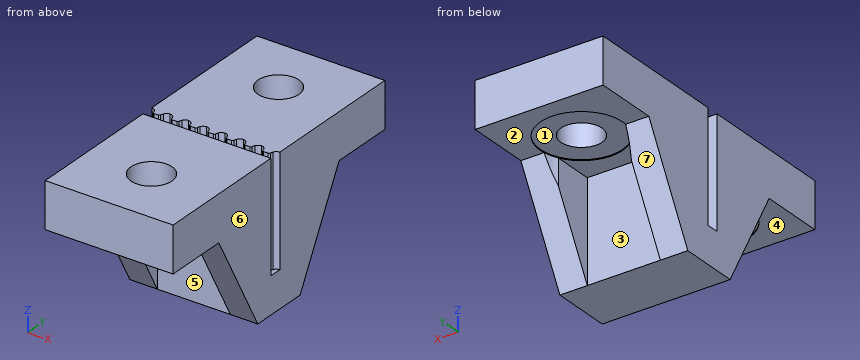
```python
from build123d import *

# Parameters (mm, degrees)
SKETCH3_W           = 14
SKETCH3_H           = 6.5
BOSS_EXTRUDE2_DEPTH = 16
CUT_EXTRUDE1_START  = 4
CUT_EXTRUDE1_DEPTH  = 19
LPATTERN2_COUNT     = 7
LPATTERN2_PITCH     = 2
SKETCH4_W           = 14
SKETCH4_H           = 13
SKETCH4_R           = 2.25
BOSS_EXTRUDE3_DEPTH = 5
BOSS_EXTRUDE4_DEPTH = 3
BOSS_EXTRUDE5_START = -11
BOSS_EXTRUDE5_DEPTH = 3
CUT_EXTRUDE2_START  = -0.1
SKETCH5_R           = 4.5
CUT_EXTRUDE2_DEPTH  = 10.1


with BuildPart() as part:
    # Sketch3 → Boss-Extrude2 (new body)
    with BuildSketch(Plane.XY):
        with Locations((7, 1.25)):
            Rectangle(SKETCH3_W, SKETCH3_H)
    extrude(amount=BOSS_EXTRUDE2_DEPTH)

    # Sketch1 → Cut-Extrude1 (cut)
    with BuildSketch(Plane.XY.offset(CUT_EXTRUDE1_START)):
        with BuildLine():
            Line((0.740175425, 0.63), (1.259824575, 0.63))
            ThreePointArc((1.259824575, 0.63), (1.358731646, 0.667228588), (1.408543109, 0.760434783))
            ThreePointArc((1.408543109, 0.760434783), (1.442388286, 0.918062154), (1.501123596, 1.068202247))
            ThreePointArc((1.501123596, 1.068202247), (1.705850588, 1.295639059), (2, 1.38))
            Line((2, 1.38), (2, 0))
            Line((2, 0), (0, 0))
            Line((0, 0), (0, 1.38))
            ThreePointArc((0, 1.38), (0.294149412, 1.295639059), (0.498876404, 1.068202247))
            ThreePointArc((0.498876404, 1.068202247), (0.557611714, 0.918062154), (0.591456891, 0.760434783))
            ThreePointArc((0.591456891, 0.760434783), (0.641268354, 0.667228588), (0.740175425, 0.63))
        make_face()
    cut_extrude1 = extrude(amount=CUT_EXTRUDE1_DEPTH, mode=Mode.SUBTRACT)

    # LPattern2: Cut-Extrude1 ×7
    with Locations(*[(i * LPATTERN2_PITCH, 0, 0) for i in range(1, LPATTERN2_COUNT)]):
        add(cut_extrude1, mode=Mode.SUBTRACT)

    # Sketch4 → Boss-Extrude3 (add)
    with BuildSketch(Plane(origin=(0, 4.5, 16), x_dir=(-1, 0, 0), z_dir=(0, 0, -1))):
        with Locations((-7, -13)):
            Rectangle(SKETCH4_W, SKETCH4_H)
        with Locations((-7, -13)):
            Circle(SKETCH4_R, mode=Mode.SUBTRACT)
        with Locations((-7, 6.5)):
            Rectangle(SKETCH4_W, SKETCH4_H)
        with Locations((-7, 6.5)):
            Circle(SKETCH4_R, mode=Mode.SUBTRACT)
    extrude(amount=BOSS_EXTRUDE3_DEPTH)

    # Sketch7 → Boss-Extrude4 (add)
    with BuildSketch(Plane.ZY):
        Polygon((0, -2), (11, -7.982839213), (11, -2), align=None)
    boss_extrude4 = extrude(amount=-BOSS_EXTRUDE4_DEPTH)

    # Sketch7_2 → Boss-Extrude5 (add)
    with BuildSketch(Plane.ZY.offset(BOSS_EXTRUDE5_START)):
        Polygon((0, -2), (11, -7.982839213), (11, -2), align=None)
    boss_extrude5 = extrude(amount=-BOSS_EXTRUDE5_DEPTH)

    # Sketch5 → Cut-Extrude2 (cut)
    with BuildSketch(Plane(origin=(0, 0, 11), x_dir=(-1, 0, 0), z_dir=(0, 0, -1)).offset(CUT_EXTRUDE2_START)):
        with Locations((-7, 11)):
            Circle(SKETCH5_R)
        with Locations((-7, -8.5)):
            Circle(SKETCH5_R)
    cut_extrude2 = extrude(amount=CUT_EXTRUDE2_DEPTH, mode=Mode.SUBTRACT)

    # Mirror1: Boss-Extrude4, Boss-Extrude5, Cut-Extrude2 across plane
    add(boss_extrude4.mirror(Plane.ZX.offset(1.25)))
    add(boss_extrude5.mirror(Plane.ZX.offset(1.25)))
    add(cut_extrude2.mirror(Plane.ZX.offset(1.25)), mode=Mode.SUBTRACT)


solid = part.part
```
The listing builds one solid part. Answer for the finished solid, in the listing's coordinates (mm). Face numbers are marked on the shaded views. A direction names the side the tool comes from. Coordinates: 2 decimals unless noted, no trailing zeros. Write each loop counter-clockwise with the first axis right and the second up, starting at its lowest first coordinate (ties: lowest second). Pieces come first, ordered by that corner, then holes. Notation, with made-up numbers: (0.5, -32.5) - (45.5, -32.5) arc R24 ccw to (45.5, -17.5) - close; hole circle Ø3 at (-10, -4.5). An arc over 180 degrees is marked (long way). Return JSON: item names as keys, results as strings. Group by question number.
Q1. The part is cut by section D-D on y = -10. Write down the section's boundary in (x, z), and give its area (3 significant figures).
Q2. Find the intervals of material crossed by line 1 along Y through (x, z) = (7, 12.7); line 2 along X through (y, z) = (7, 9); line 3 along Y through (x, z) = (7, 9.65), in increasing order. Write a range as [from, to].
Q3. Which of the six approach directions +Z, -Z, +X, -X, +Y, -Y give full straight-line access (tool end or side, diameter ignored) to the marked faces 1, 2, 3 and 4?
Q4. The part is cut by section A-A on y = 11. Write down the section's boundary in (x, z).
Q5. The part is cut by section C-C on y = -3. Write down the section's boundary in (x, z), and give its area (3 significant figures).
Q6. Flat-ended cylindrical pins translate along their axes: pin 1 Ø3.5 at (x, y) = (9, -4.5) entering from -Z; pin 2 Ø6.5 at (x, z) = (7.5, 5) entering from -Y; pin 3 Ø4 at (y, z) = (-7.5, 3) entering from -X; pin 4 Ø5 at (y, z) = (-4.5, 3) entering from -X. Find the tip coordinate at first contact, or state that the pin passes through.
Q7. The part is cut by section B-B on z = 15.25. State how many separate pieces and enclosed holes the cut face has, and give its area (3 significant figures).
Q8. For a pull along X with two mould halves and no side action, classify the marked faces 5, 6 and 7 as +X half, -X half, draft (parallel to the pull), parting line (faces both ways), or undercut.
Evaluation:
{
 "1": {"outline": "(0, 11) - (2.76, 11) - (2.76, 11.1) - (5.32, 11.1) - (5.32, 16) - (0, 16) - close; (8.68, 11.1) - (11.24, 11.1) - (11.24, 11) - (14, 11) - (14, 16) - (8.68, 16) - close", "area": "52.7 mm2"},
 "2": {"line 1": "y = [-15, -10.75], [-6.25, 0], [0.63, 8.75], [13.25, 17.5]", "line 2": "x = [0, 3], [11, 14]", "line 3": "y = [-2, 0], [0.63, 4.5]"},
 "3": {"face 1": "-Z", "face 2": "-Z, +X, -X, +Y", "face 3": "-Z, +Y", "face 4": "-Z, +X, -X, -Y"},
 "4": {"outline": "(0, 11) - (2.5, 11) - (2.5, 11.1) - (4.75, 11.1) - (4.75, 16) - (0, 16) - close; (9.25, 11.1) - (11.5, 11.1) - (11.5, 11) - (14, 11) - (14, 16) - (9.25, 16) - close"},
 "5": {"outline": "(0, 1.84) - (3, 1.84) - (3, 11) - (11, 11) - (11, 1.84) - (14, 1.84) - (14, 16) - (0, 16) - close", "area": "125 mm2"},
 "6": {"pin 1": "stops at z = 11", "pin 2": "stops at y = -2", "pin 3": "passes through", "pin 4": "stops at x = 0"},
 "7": {"separate pieces": "2", "enclosed holes": "2", "area": "409 mm2"},
 "8": {"face 5": "undercut", "face 6": "+X half", "face 7": "draft"}
}
